Input: dimensioned drawing with shaded views. Units: mm. Origin: part minimum x, y, z. A direction names the side the tool comes from. Give positions to 0.01 mm unless a question says otherwise; leave off trailing zeros. Loops run counter-clockwise (first coordinate to the right, second up) from the corner with the lowest first, then second, coordinate; pieces in that order, holes last.
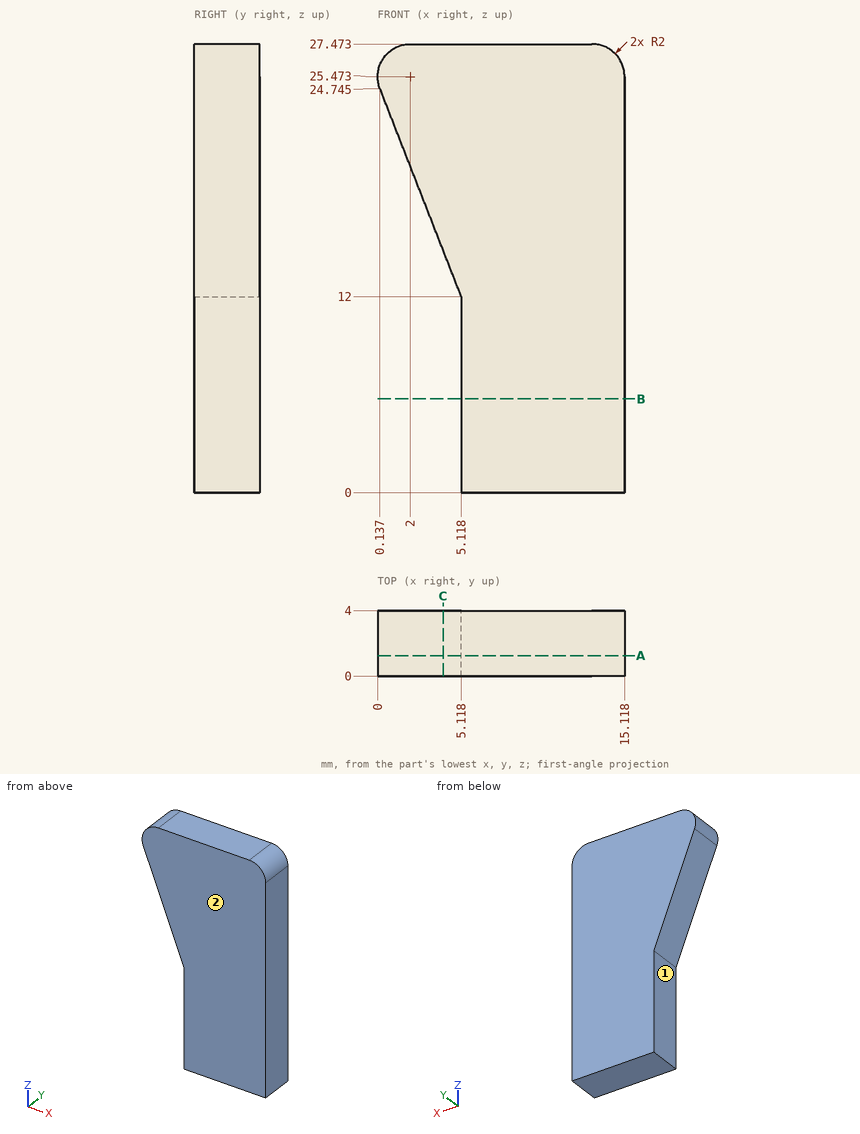
Item 1: Section query A-A on y = 1.25. Return loops of the section in (x, z) (1 decimal), plus the area to 3 significant figures.
Values follow:
outline: (0.1, 24.7) - (5.1, 12) - (5.1, 0) - (15.1, 0) - (15.1, 25.5) arc R2 ccw to (13.1, 27.5) - (2, 27.5) arc R2 ccw to start
area: 319 mm2
Item 2: Section query C-C on x = 4. Return loops of the section in (y, z).
Values follow:
outline: (0, 14.86) - (4, 14.86) - (4, 27.47) - (0, 27.47) - close
Item 3: Ray query, probe 1 along X at (y, z) = (1.6, 6.5); probe 2 along X at (y, z) = (1.7, 13.75) (1 decimal). Return the intervals inside material, ascending.
Values follow:
probe 1: x = 5.12 to 15.12
probe 2: x = 4.4 to 15.1
Item 4: Section query B-B on z = 5.75. Return loops of the section in (x, y), plus the area to 3 significant figures.
Values follow:
outline: (5.12, 0) - (15.12, 0) - (15.12, 4) - (5.12, 4) - close
area: 40.0 mm2
Item 5: Set-up query: the marked faces 1 and 2. Return all of +Z, -Z, +X, -X, +Y, -Y with unobstructed straight access to the full face (end or side cutting, diameter ignored); none if empty.
Values follow:
face 1: -Z, -X, +Y, -Y
face 2: +Z, -Z, +X, -X, -Y
